from build123d import *

# Parameters (mm, degrees)
SKETCH2_W                     = 59
SKETCH2_H                     = 25
BOSS_EXTRUDE1_DEPTH           = 1.5875
EDGE_FLANGE2_STRIP_W          = 9.525
EDGE_FLANGE2_STRIP_H          = 1.5875
EDGE_FLANGE2_STRIP_CUT_DEPTH  = 9.5
EDGE_FLANGE2_RELIEF_W         = 10.31875
EDGE_FLANGE2_RELIEF_H         = 0.79375
EDGE_FLANGE2_RELIEF_CUT_DEPTH = 1.5875
EDGE_FLANGE2_DEPTH            = 9.5
EDGE_FLANGE3_STRIP_W          = 9.525
EDGE_FLANGE3_STRIP_H          = 1.5875
EDGE_FLANGE3_STRIP_CUT_DEPTH  = 9.5
EDGE_FLANGE3_RELIEF_W         = 10.31875
EDGE_FLANGE3_RELIEF_H         = 0.79375
EDGE_FLANGE3_RELIEF_CUT_DEPTH = 1.5875
EDGE_FLANGE3_DEPTH            = 9.5
CUT_EXTRUDE1_REACH            = 69.127
SKETCH16_R                    = 1
SKETCH18_W                    = 38.4125
SKETCH18_H                    = 12
BOSS_EXTRUDE2_DEPTH           = 1.5875
SKETCH19_R                    = 1.5
SKETCH19_W                    = 9.5
SKETCH19_H                    = 3.825
CUT_EXTRUDE2_DEPTH            = 1.5875
EDGE_FLANGE4_STRIP_W          = 9.525
EDGE_FLANGE4_STRIP_H          = 1.5875
EDGE_FLANGE4_STRIP_CUT_DEPTH  = 40
EDGE_FLANGE4_DEPTH            = 40
FILLET1_R                     = 2
SKETCH24_W                    = 38.4125
SKETCH24_H                    = 15.96875
CUT_EXTRUDE3_DEPTH            = 10


# Sheet-metal steps are written as plain solids
with BuildPart() as part:
    # Sketch2 → Boss-Extrude1 (new body)
    with BuildSketch(Plane(origin=(0, 0, 0), x_dir=(1, 0, 0), z_dir=(0, 1, 0))):
        with Locations((29.5, 12.5)):
            Rectangle(SKETCH2_W, SKETCH2_H)
    extrude(amount=BOSS_EXTRUDE1_DEPTH)

    # Edge-Flange2 strip (across the edge) → Edge-Flange2 strip cut (cut)
    with BuildSketch(Plane(origin=(59, 1.5875, -25), x_dir=(0, 0, 1), z_dir=(-1, 0, 0))):
        with Locations((-1.5875, -0.79375)):
            Rectangle(EDGE_FLANGE2_STRIP_W, EDGE_FLANGE2_STRIP_H)
    extrude(amount=EDGE_FLANGE2_STRIP_CUT_DEPTH, mode=Mode.SUBTRACT)

    # Edge-Flange2 relief (on the sheet) → Edge-Flange2 relief cut (cut)
    with BuildSketch(Plane(origin=(59, 1.5875, -21.825), x_dir=(0, 0, 1), z_dir=(0, 1, 0))):
        with Locations((-4.365625, -9.896875)):
            Rectangle(EDGE_FLANGE2_RELIEF_W, EDGE_FLANGE2_RELIEF_H)
    extrude(amount=-EDGE_FLANGE2_RELIEF_CUT_DEPTH, mode=Mode.SUBTRACT)

    # Edge-Flange2 section (across the edge) → Edge-Flange2 (add)
    with BuildSketch(Plane(origin=(59, 1.5875, -25), x_dir=(0, 0, 1), z_dir=(-1, 0, 0))):
        with BuildLine():
            Line((0, 1.5875), (0, 18.4125))
            Line((0, 18.4125), (1.5875, 18.4125))
            Line((1.5875, 18.4125), (1.5875, 1.5875))
            ThreePointArc((1.5875, 1.5875), (2.052467985, 0.464967985), (3.175, 0))
            Line((3.175, 0), (3.175, -1.5875))
            ThreePointArc((3.175, -1.5875), (0.92993597, -0.65756403), (0, 1.5875))
        make_face()
    extrude(amount=EDGE_FLANGE2_DEPTH)

    # Edge-Flange3 strip (across the edge) → Edge-Flange3 strip cut (cut)
    with BuildSketch(Plane(origin=(9.5, 1.5875, -25), x_dir=(0, 0, 1), z_dir=(-1, 0, 0))):
        with Locations((-1.5875, -0.79375)):
            Rectangle(EDGE_FLANGE3_STRIP_W, EDGE_FLANGE3_STRIP_H)
    extrude(amount=EDGE_FLANGE3_STRIP_CUT_DEPTH, mode=Mode.SUBTRACT)

    # Edge-Flange3 relief (on the sheet) → Edge-Flange3 relief cut (cut)
    with BuildSketch(Plane(origin=(9.5, 1.5875, -21.825), x_dir=(0, 0, 1), z_dir=(0, 1, 0))):
        with Locations((-4.365625, 0.396875)):
            Rectangle(EDGE_FLANGE3_RELIEF_W, EDGE_FLANGE3_RELIEF_H)
    extrude(amount=-EDGE_FLANGE3_RELIEF_CUT_DEPTH, mode=Mode.SUBTRACT)

    # Edge-Flange3 section (across the edge) → Edge-Flange3 (add)
    with BuildSketch(Plane(origin=(9.5, 1.5875, -25), x_dir=(0, 0, 1), z_dir=(-1, 0, 0))):
        with BuildLine():
            Line((0, 1.5875), (0, 18.4125))
            Line((0, 18.4125), (1.5875, 18.4125))
            Line((1.5875, 18.4125), (1.5875, 1.5875))
            ThreePointArc((1.5875, 1.5875), (2.052467985, 0.464967985), (3.175, 0))
            Line((3.175, 0), (3.175, -1.5875))
            ThreePointArc((3.175, -1.5875), (0.92993597, -0.65756403), (0, 1.5875))
        make_face()
    extrude(amount=EDGE_FLANGE3_DEPTH)

    # Sketch16 → Cut-Extrude1 (cut, up to next)
    with BuildSketch(Plane(origin=(0, 0, -25), x_dir=(-1, 0, 0), z_dir=(0, 0, -1)), mode=Mode.PRIVATE) as cut_extrude1_sk1:
        with Locations(Location((-54.25, 16.5875, 0), (0, 0, 90))):
            Circle(SKETCH16_R)
    cut_extrude1_tool1 = extrude(cut_extrude1_sk1.sketch, amount=-CUT_EXTRUDE1_REACH, mode=Mode.PRIVATE) & part.part
    # Sketch16 → Cut-Extrude1 (cut, up to next)
    with BuildSketch(Plane(origin=(0, 0, -25), x_dir=(-1, 0, 0), z_dir=(0, 0, -1)), mode=Mode.PRIVATE) as cut_extrude1_sk2:
        with Locations(Location((-54.25, 6.5875, 0), (0, 0, 90))):
            Circle(SKETCH16_R)
    cut_extrude1_tool2 = extrude(cut_extrude1_sk2.sketch, amount=-CUT_EXTRUDE1_REACH, mode=Mode.PRIVATE) & part.part
    # Sketch16 → Cut-Extrude1 (cut, up to next)
    with BuildSketch(Plane(origin=(0, 0, -25), x_dir=(-1, 0, 0), z_dir=(0, 0, -1)), mode=Mode.PRIVATE) as cut_extrude1_sk3:
        with Locations(Location((-4.75, 6.5875, 0), (0, 0, 270))):
            Circle(SKETCH16_R)
    cut_extrude1_tool3 = extrude(cut_extrude1_sk3.sketch, amount=-CUT_EXTRUDE1_REACH, mode=Mode.PRIVATE) & part.part
    # Sketch16 → Cut-Extrude1 (cut, up to next)
    with BuildSketch(Plane(origin=(0, 0, -25), x_dir=(-1, 0, 0), z_dir=(0, 0, -1)), mode=Mode.PRIVATE) as cut_extrude1_sk4:
        with Locations(Location((-4.75, 16.5875, 0), (0, 0, 270))):
            Circle(SKETCH16_R)
    cut_extrude1_tool4 = extrude(cut_extrude1_sk4.sketch, amount=-CUT_EXTRUDE1_REACH, mode=Mode.PRIVATE) & part.part
    add(cut_extrude1_tool1.solids().sort_by_distance((54.25, 16.5875, -25))[0], mode=Mode.SUBTRACT)
    add(cut_extrude1_tool2.solids().sort_by_distance((54.25, 6.5875, -25))[0], mode=Mode.SUBTRACT)
    add(cut_extrude1_tool3.solids().sort_by_distance((4.75, 6.5875, -25))[0], mode=Mode.SUBTRACT)
    add(cut_extrude1_tool4.solids().sort_by_distance((4.75, 16.5875, -25))[0], mode=Mode.SUBTRACT)

    # Sketch18 → Boss-Extrude2 (add)
    with BuildSketch(Plane(origin=(0, 1.5875, 0), x_dir=(1, 0, 0), z_dir=(0, 1, 0))):
        with Locations((29.5, 31)):
            Rectangle(SKETCH18_W, SKETCH18_H)
    extrude(amount=-BOSS_EXTRUDE2_DEPTH)

    # Sketch19 → Cut-Extrude2 (cut)
    with BuildSketch(Plane(origin=(0, 1.5875, 0), x_dir=(1, 0, 0), z_dir=(0, 1, 0))):
        with Locations(Location((4.75, 17.825, 0), (0, 0, 270))):
            Circle(SKETCH19_R)
        with Locations(Location((4.75, 7.825, 0), (0, 0, 270))):
            Circle(SKETCH19_R)
        with Locations(Location((54.25, 17.825, 0), (0, 0, 90))):
            Circle(SKETCH19_R)
        with Locations(Location((54.25, 7.825, 0), (0, 0, 90))):
            Circle(SKETCH19_R)
        with Locations((54.25, 1.9125)):
            Rectangle(SKETCH19_W, SKETCH19_H)
        with Locations((4.75, 1.9125)):
            Rectangle(SKETCH19_W, SKETCH19_H)
    extrude(amount=-CUT_EXTRUDE2_DEPTH, mode=Mode.SUBTRACT)

    # Edge-Flange4 strip (across the edge) → Edge-Flange4 strip cut (cut)
    with BuildSketch(Plane(origin=(9.5, 1.5875, 0), x_dir=(0, 0, -1), z_dir=(1, 0, 0))):
        with Locations((-3.175, -0.79375)):
            Rectangle(EDGE_FLANGE4_STRIP_W, EDGE_FLANGE4_STRIP_H)
    extrude(amount=EDGE_FLANGE4_STRIP_CUT_DEPTH, mode=Mode.SUBTRACT)

    # Edge-Flange4 section (across the edge) → Edge-Flange4 (add)
    with BuildSketch(Plane(origin=(9.5, 1.5875, 0), x_dir=(0, 0, -1), z_dir=(1, 0, 0))):
        with BuildLine():
            Line((-1.5875, 1.5875), (-1.5875, 18.4125))
            Line((-1.5875, 18.4125), (0, 18.4125))
            Line((0, 18.4125), (0, 1.5875))
            ThreePointArc((0, 1.5875), (0.464967985, 0.464967985), (1.5875, 0))
            Line((1.5875, 0), (1.5875, -1.5875))
            ThreePointArc((1.5875, -1.5875), (-0.65756403, -0.65756403), (-1.5875, 1.5875))
        make_face()
    extrude(amount=EDGE_FLANGE4_DEPTH)

    # Fillet1
    fillet1_edges = [part.edges().sort_by_distance(p)[0] for p in [
        (10.29375, 0.79375, -37),
        (48.70625, 0.79375, -37),
        (0, 0.79375, -3.825),
        (59, 0.79375, -3.825),
        (9.5, 20, 0.79375),
        (49.5, 20, 0.79375),
        (59, 20, -24.20625),
        (49.5, 20, -24.20625),
        (9.5, 20, -24.20625),
        (0, 20, -24.20625),
    ]]
    fillet(fillet1_edges, radius=FILLET1_R)

    # Sketch24 → Cut-Extrude3 (cut)
    with BuildSketch(Plane(origin=(0, 1.5875, 0), x_dir=(1, 0, 0), z_dir=(0, 1, 0))):
        with Locations((29.5, 29.015625)):
            Rectangle(SKETCH24_W, SKETCH24_H)
    extrude(amount=-CUT_EXTRUDE3_DEPTH, mode=Mode.SUBTRACT)


solid = part.part
Input: part model. Units: mm. Frame: model coordinates. A direction names the side the tool comes from. Give positions to 0.01 mm unless a question says otherwise; leave off trailing zeros. Loops run counter-clockwise (first coordinate to the right, second up) from the corner with the lowest first, then second, coordinate; pieces in that order, holes last. Notation, with made-up numbers: (10, -14) - (58, -14) arc R35 ccw to (58, 21) - close; hole circle Ø2 at (-22.75, 70.5). An arc over 180 degrees is marked (long way). Use CSV: the item, a comma, the result in double quotes. Start each with the question number.
Item 1: Mould query, pull axis X, two halves, no side actions, for faces 1 (the cylindrical face through (0.57, 19.4, -24.2)), 2 (the flat face through (54, 12, -23.412)), 3 (the cylindrical face through (55.163, 0.805, -6.635)). Classes: pulls with the +X half, pulls with the -X half, needs draft (parallel to the pull), parting line crosses it, or undercut.
Item 2: Section A-A on y = 14.25. Return loops of the section in (x, z).
Item 3: Section B-B on x = 4.75. State how many separate pieces and enclosed holes the cut face has, then the cut area to 3 significant figures.
Item 4: Section C-C on z = -8.25. Return loops of the section in (x, y).
Item 5: Line query: line 1 (Y direction, x = 23, z = -3); line 2 (Z direction, x = 8, y = 18). Output: solid intervals per line, ascending.
Item 6: Reachability of faces 4 (the flat face through (29, 1.588, -12)), 5 (the flat face through (9.5, 7, 1)), 6 (the flat face through (49.5, 7, 1)) from +Z, -Z, +X, -X, +Y, -Y: full face, straight path, thin tool, end or side. Return the list, or none.
Item 7: Contact query for flat-ended pins moving along their axis: P1, Ø2.5, axis at x = 4.75, y = 6.59, coming from the +Z side; P2, Ø1.3, axis at x = 52.5, y = 1, coming from the +Z side (3 decimals); P3, Ø8, axis at y = 17.5, z = -3, coming from the -X side. Output: stop coordinate, or through.
Ans:
1,face 1,"pulls with the -X half"
1,face 2,"needs draft"
1,face 3,"undercut"
2,outline,"(0, -25) - (9.5, -25) - (9.5, -23.41) - (0, -23.41) - close; (9.5, 0) - (49.5, 0) - (49.5, 1.59) - (9.5, 1.59) - close; (49.5, -25) - (59, -25) - (59, -23.41) - (49.5, -23.41) - close"
3,separate pieces,"5"
3,enclosed holes,"0"
3,area,"45.3 mm2"
4,outline,"(0, 0) - (3.31, 0) - (3.31, 1.59) - (0, 1.59) - close; (6.19, 0) - (52.81, 0) - (52.81, 1.59) - (6.19, 1.59) - close; (55.69, 0) - (59, 0) - (59, 1.59) - (55.69, 1.59) - close"
5,line 1,"y = 0 to 1.59"
5,line 2,"z = -25 to -23.41"
6,face 4,"+X, -X, +Y"
6,face 5,"+Z, -X, +Y, -Y"
6,face 6,"+Z, +X, +Y, -Y"
7,P1,"stops at z = -23.41"
7,P2,"stops at z = -3.825"
7,P3,"stops at x = 9.5"
